Geometry: final body of the model. Coordinates: model frame, mm. A direction names the side the tool comes from. Give positions to 0.01 mm unless a question says otherwise; leave off trailing zeros. Loops run counter-clockwise (first coordinate to the right, second up) from the corner with the lowest first, then second, coordinate; pieces in that order, holes last.
Autodesk Inventor part; units mm, degrees
ref_plane "YZ Plane" through (0, 0, 0) normal (1, 0, 0) x (0, 1, 0)
ref_plane "XZ Plane" through (0, 0, 0) normal (0, 1, 0) x (-1, 0, 0)
ref_plane "XY Plane" through (0, 0, 0) normal (0, 0, 1) x (1, 0, 0)
sketch "Sketch1" plane through (0, 0, 0) normal (0, 1, 0) x (-1, 0, 0)
  line L0 (56.896, 29.845) -> (-56.896, 29.845)
  line L1 (-56.896, 29.845) -> (-56.896, -29.845)
  line L2 (-56.896, -29.845) -> (56.896, -29.845)
  line L3 (56.896, -29.845) -> (56.896, 29.845)
  line L4 (56.896, 29.845) -> (-56.896, -29.845) construction
  line L5 (-56.896, 29.845) -> (56.896, -29.845) construction
  line L6 (57.896, -30.845) -> (-57.896, -30.845)
  line L7 (-57.896, -30.845) -> (-57.896, 30.845)
  line L8 (-57.896, 30.845) -> (57.896, 30.845)
  line L9 (57.896, 30.845) -> (57.896, -30.845)
  point P0 (0, 0)
  dimension "d0" = 113.792
  dimension "d1" = 59.69
  dimension "d2" = 1
extrude "Extrusion1" add sketch "Sketch1" along normal blind 6.35
properties part number "band" material "Rubber"
Item 1: Draft query along Z for faces 3 (the face through (1, 3, 30.845)), 4 (the face through (-56.896, 3, 0)), 5 (the face through (-1, 3, 29.845)), 6 (the face through (0, 6.35, 30)). Return one class per face: +Z half, -Z half, draft (parallel to the pull), parting line (faces both ways), or undercut.
Values follow:
face 3: +Z half
face 4: undercut
face 5: undercut
face 6: draft
Item 2: Section query B-B on y = 1.75. Return loops of the section in (x, z) (3 decimals), plus the area to 3 significant figures.
Values follow:
outline: (-57.896, -30.845) - (57.896, -30.845) - (57.896, 30.845) - (-57.896, 30.845) - close; hole (-56.896, -29.845) - (56.896, -29.845) - (56.896, 29.845) - (-56.896, 29.845) - close
area: 351 mm2
Item 3: Section query C-C on x = -45.5. Return loops of the section in (y, z) (3 decimals), plus the area to 3 significant figures.
Values follow:
outline: (0, -30.845) - (6.35, -30.845) - (6.35, -29.845) - (0, -29.845) - close; (0, 29.845) - (6.35, 29.845) - (6.35, 30.845) - (0, 30.845) - close
area: 12.7 mm2
Item 4: Set-up query: faces 1 (the face through (1, 3, -29.845)), 2 (the face through (-1, 3, -30.845)). Return all of +Z, -Z, +X, -X, +Y, -Y with unobstructed straight access to the full face (end or side cutting, diameter ignored); none if empty.
Values follow:
face 1: +Y, -Y
face 2: -Z, +X, -X, +Y, -Y
Item 5: Ray query, probe 1 along X at (y, z) = (3, -21.5); probe 2 along Z at (x, y) = (32, 6.25) (3 decimals). Return the intervals inside material, ascending.
Values follow:
probe 1: x = -57.9 to -56.9, 56.9 to 57.9
probe 2: z = -30.845 to -29.845, 29.845 to 30.845
Item 6: Section query A-A on z = -23. Return loops of the section in (x, y), plus the area to 3 significant figures.
Values follow:
outline: (-57.9, 0) - (-56.9, 0) - (-56.9, 6.35) - (-57.9, 6.35) - close; (56.9, 0) - (57.9, 0) - (57.9, 6.35) - (56.9, 6.35) - close
area: 12.7 mm2
